CAD build for the part. Positions are in the model's coordinates, mm. Face numbers are marked on the shaded views. A direction names the side the tool comes from. Give positions to 0.01 mm unless a question says otherwise; leave off trailing zeros. Write each loop counter-clockwise with the first axis right and the second up, starting at its lowest first coordinate (ties: lowest second). Pieces come first, ordered by that corner, then holes. Notation, with made-up numbers: (73.5, 84) -> (108.5, 84) arc R27 ccw to (108.5, 118) -> close; hole circle Ø4 at (-34, -11). An arc over 180 degrees is marked (long way). Answer as a JSON object with one key per item and string values.
```python
from build123d import *

# Parameters (mm, degrees)
SKETCH_1_R          = 4.5
SKETCH_1_R_2        = 3
EXTRUDE_1_DEPTH     = 10
EXTRUDE_2_DEPTH     = 16
SKETCH_3_R          = 1.5
EXTRUDE_3_DEPTH     = 10
SKETCH_5_W          = 16
SKETCH_5_H          = 32
CUT_EXTRUDE_1_DEPTH = 0.1
SKETCH_6_W          = 32
SKETCH_6_H          = 16
CUT_EXTRUDE_2_DEPTH = 0.1
SKETCH_7_W          = 16
SKETCH_7_H          = 32
CUT_EXTRUDE_3_DEPTH = 0.1
SKETCH_8_W          = 32
SKETCH_8_H          = 16
CUT_EXTRUDE_4_DEPTH = 0.1
SKETCH_9_R          = 1.5
CUT_EXTRUDE_5_DEPTH = 40.471508712
SKETCH_10_R         = 11
EXTRUDE_4_DEPTH     = 1.5
CUT_EXTRUDE_START   = -3
SKETCH_11_R         = 4.5
CUT_EXTRUDE_6_DEPTH = 3
SKETCH_12_R         = 4
EXTRUDE_5_DEPTH     = 9
CHAMFER_1_SIZE      = 1
SKETCH_13_R         = 2.5
EXTRUDE_6_DEPTH     = 21
CUT_EXTRUDE_START_2 = -0.1
SKETCH_14_R         = 2.8
SKETCH_14_R_2       = 2.5
CUT_EXTRUDE_7_DEPTH = 0.1
SKETCH_15_R         = 4.5
SKETCH_15_R_2       = 4.3
CUT_EXTRUDE_8_DEPTH = 0.1
CHAMFER_2_SIZE      = 0.5


with BuildPart() as part:
    # 草图1 → 凸台-拉伸1 (new body)
    with BuildSketch(Plane.XY):
        Polygon((-21, 17), (-17, 21), (17, 21), (21, 17), (21, -17), (17, -21), (-17, -21), (-21, -17), align=None)
        Circle(SKETCH_1_R, mode=Mode.SUBTRACT)
        with Locations((-16, 16)):
            Circle(SKETCH_1_R_2, mode=Mode.SUBTRACT)
        with Locations(Location((16, 16, 0), (0, 0, 180))):
            Circle(SKETCH_1_R_2, mode=Mode.SUBTRACT)
        with Locations((16, -16)):
            Circle(SKETCH_1_R_2, mode=Mode.SUBTRACT)
        with Locations(Location((-16, -16, 0), (0, 0, 180))):
            Circle(SKETCH_1_R_2, mode=Mode.SUBTRACT)
    extrude(amount=EXTRUDE_1_DEPTH)

    # 草图2 → 凸台-拉伸2 (add)
    with BuildSketch(Plane.XY.offset(10)):
        Polygon((16, 21), (-16, 21), (-21, 16), (-21, -16), (-16, -21), (16, -21), (21, -16), (21, 16), align=None)
    extrude(amount=EXTRUDE_2_DEPTH)

    # 草图3 → 凸台-拉伸3 (add)
    with BuildSketch(Plane.XY.offset(26)):
        Polygon((-17, 21), (-21, 17), (-21, 16), (-21, -16), (-21, -17), (-17, -21), (-16, -21), (16, -21), (17, -21), (21, -17), (21, -16), (21, 16), (21, 17), (17, 21), (16, 21), (-16, 21), align=None)
        with Locations((-16, 16)):
            Circle(SKETCH_3_R, mode=Mode.SUBTRACT)
        with Locations(Location((16, 16, 0), (0, 0, 180))):
            Circle(SKETCH_3_R, mode=Mode.SUBTRACT)
        with Locations((16, -16)):
            Circle(SKETCH_3_R, mode=Mode.SUBTRACT)
        with Locations(Location((-16, -16, 0), (0, 0, 180))):
            Circle(SKETCH_3_R, mode=Mode.SUBTRACT)
    extrude(amount=EXTRUDE_3_DEPTH)

    # 草图5 → 切除-拉伸1 (cut)
    with BuildSketch(Plane.ZY.offset(21)):
        with Locations((18, 0)):
            Rectangle(SKETCH_5_W, SKETCH_5_H)
    extrude(amount=-CUT_EXTRUDE_1_DEPTH, mode=Mode.SUBTRACT)

    # 草图6 → 切除-拉伸2 (cut)
    with BuildSketch(Plane(origin=(0, 21, 0), x_dir=(1, 0, 0), z_dir=(0, 1, 0))):
        with Locations((0, -18)):
            Rectangle(SKETCH_6_W, SKETCH_6_H)
    extrude(amount=-CUT_EXTRUDE_2_DEPTH, mode=Mode.SUBTRACT)

    # 草图7 → 切除-拉伸3 (cut)
    with BuildSketch(Plane(origin=(21, 0, 0), x_dir=(0, 0, -1), z_dir=(1, 0, 0))):
        with Locations((-18, 0)):
            Rectangle(SKETCH_7_W, SKETCH_7_H)
    extrude(amount=-CUT_EXTRUDE_3_DEPTH, mode=Mode.SUBTRACT)

    # 草图8 → 切除-拉伸4 (cut)
    with BuildSketch(Plane.XZ.offset(21)):
        with Locations((0, 18)):
            Rectangle(SKETCH_8_W, SKETCH_8_H)
    extrude(amount=-CUT_EXTRUDE_4_DEPTH, mode=Mode.SUBTRACT)

    # 草图9 → 切除-拉伸5 (cut, through all)
    with BuildSketch(Plane.XY.offset(26)):
        with Locations(Location((-16, -16, 0), (0, 0, 180))):
            Circle(SKETCH_9_R)
        with Locations((-16, 16)):
            Circle(SKETCH_9_R)
        with Locations(Location((16, 16, 0), (0, 0, 180))):
            Circle(SKETCH_9_R)
        with Locations((16, -16)):
            Circle(SKETCH_9_R)
    extrude(amount=-CUT_EXTRUDE_5_DEPTH, mode=Mode.SUBTRACT)

    # 草图10 → 凸台-拉伸4 (add)
    with BuildSketch(Plane.XY.offset(36)):
        Circle(SKETCH_10_R)
    extrude(amount=EXTRUDE_4_DEPTH)

    # 草图11 → 切除-拉伸6 (cut)
    with BuildSketch(Plane.XY.offset(37.5).offset(CUT_EXTRUDE_START)):
        Circle(SKETCH_11_R)
    extrude(amount=CUT_EXTRUDE_6_DEPTH, mode=Mode.SUBTRACT)

    # 草图12 → 凸台-拉伸5 (add)
    with BuildSketch(Plane(origin=(0, 0, 10), x_dir=(-1, 0, 0), z_dir=(0, 0, -1))):
        with Locations(Location((0, 0, 0), (0, 0, 180))):
            Circle(SKETCH_12_R)
    extrude(amount=EXTRUDE_5_DEPTH)

    # 倒角1
    chamfer_1_edges = [part.edges().sort_by_distance(p)[0] for p in [
        (-4, 0, 1),
    ]]
    chamfer(chamfer_1_edges, length=CHAMFER_1_SIZE)

    # 草图13 → 凸台-拉伸6 (add)
    with BuildSketch(Plane.XY.offset(34.5)):
        with Locations(Location((0, 0, 0), (0, 0, 180))):
            Circle(SKETCH_13_R)
    extrude(amount=EXTRUDE_6_DEPTH)

    # 草图14 → 切除-拉伸7 (cut)
    with BuildSketch(Plane.XY.offset(34.5).offset(CUT_EXTRUDE_START_2)):
        Circle(SKETCH_14_R)
        with Locations(Location((0, 0, 0), (0, 0, 180))):
            Circle(SKETCH_14_R_2, mode=Mode.SUBTRACT)
    extrude(amount=CUT_EXTRUDE_7_DEPTH, mode=Mode.SUBTRACT)

    # 草图15 → 切除-拉伸8 (cut)
    with BuildSketch(Plane.XY.offset(34.5).offset(CUT_EXTRUDE_START_2)):
        Circle(SKETCH_15_R)
        Circle(SKETCH_15_R_2, mode=Mode.SUBTRACT)
    extrude(amount=CUT_EXTRUDE_8_DEPTH, mode=Mode.SUBTRACT)

    # 倒角2
    chamfer_2_edges = [part.edges().sort_by_distance(p)[0] for p in [
        (2.5, 0, 55.5),
    ]]
    chamfer(chamfer_2_edges, length=CHAMFER_2_SIZE)


solid = part.part
```
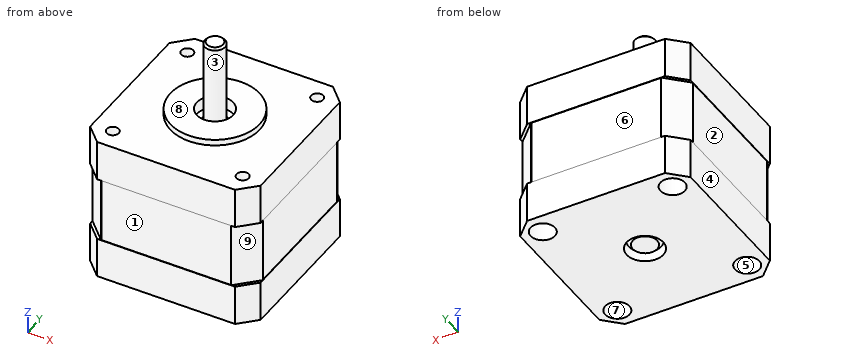
1) Slice it at B-B (x = -8.5). List the corners of the cut face in (y, z), then the cut area to 3 significant figures.
Model answer:
{"outline": "(-21, 0) -> (21, 0) -> (21, 10) -> (20.9, 10) -> (20.9, 26) -> (21, 26) -> (21, 36) -> (6.98, 36) -> (6.98, 37.5) -> (-6.98, 37.5) -> (-6.98, 36) -> (-21, 36) -> (-21, 26) -> (-20.9, 26) -> (-20.9, 10) -> (-21, 10) -> close", "area": "1,530 mm2"}
2) Slice it at D-D (y = 9). List the corners of the cut face in (x, z), then the cut area to 3 significant figures.
Model answer:
{"outline": "(-21, 0) -> (21, 0) -> (21, 10) -> (20.9, 10) -> (20.9, 26) -> (21, 26) -> (21, 36) -> (6.32, 36) -> (6.32, 37.5) -> (-6.32, 37.5) -> (-6.32, 36) -> (-21, 36) -> (-21, 26) -> (-20.9, 26) -> (-20.9, 10) -> (-21, 10) -> close", "area": "1,530 mm2"}
3) Mould opens along Z. For the marked faces 6, 7, 8 and 9 say: released by +Z, released by -Z, zero draft, split by the parting line, or undercut.
Model answer:
{"face 6": "undercut", "face 7": "zero draft", "face 8": "released by +Z", "face 9": "undercut"}
4) 3-axis set-ups, long thin cutter, end or side, ignore diameter. For the marked faces 1, 2, 3, 4 and 5: which of +Z, -Z, +X, -X, +Y, -Y reach the whole face in a straight line?
Model answer:
{"face 1": "-Y", "face 2": "-X", "face 3": "+Z", "face 4": "+Z, -Z, -X, +Y, -Y", "face 5": "-Z"}
5) Wall check: probe 1 along Y at (x, z) = (16, 30); probe 2 along Y at (x, z) = (0, 5); probe 3 along X at (y, z) = (15.5, 25). Give the ranges that are in metal, low to high.
Model answer:
{"probe 1": "y = -21 to -17.5, -14.5 to 14.5, 17.5 to 21", "probe 2": "y = -21 to -4.5, -4 to 4, 4.5 to 21", "probe 3": "x = -20.9 to -17.41, -14.59 to 14.59, 17.41 to 20.9"}
6) Slice it at A-A (z = 33). List the corners of the cut face in (x, y), then the cut area to 3 significant figures.
Model answer:
{"outline": "(-21, -17) -> (-17, -21) -> (17, -21) -> (21, -17) -> (21, 17) -> (17, 21) -> (-17, 21) -> (-21, 17) -> close; hole circle Ø3 at (-16, -16); hole circle Ø3 at (-16, 16); hole circle Ø3 at (16, -16); hole circle Ø3 at (16, 16)", "area": "1,700 mm2"}
7) Pin check, flat tips, straight feed: pin 1 (2.5 mm diameter, centred on x = 19.5, y = -19, fed in from +Z); pin 2 (1.5 mm diameter, centred on y = 2.5, z = 17.5, fed in from +X); pin 3 (1.8 mm diameter, centred on x = -15, y = -15.5, fed in from -Z). Stop position of each tip, or through.
Model answer:
{"pin 1": "stops at z = 36", "pin 2": "stops at x = 20.9", "pin 3": "stops at z = 10"}
8) Slice it at C-C (z = 23.5). List the corners of the cut face in (x, y).
Model answer:
{"outline": "(-21, -16) -> (-16, -21) -> (-16, -20.9) -> (16, -20.9) -> (16, -21) -> (21, -16) -> (20.9, -16) -> (20.9, 16) -> (21, 16) -> (16, 21) -> (16, 20.9) -> (-16, 20.9) -> (-16, 21) -> (-21, 16) -> (-20.9, 16) -> (-20.9, -16) -> close; hole circle Ø3 at (-16, -16); hole circle Ø3 at (-16, 16); hole circle Ø3 at (16, -16); hole circle Ø3 at (16, 16)"}
